CAD build for the part. Positions are in the model's coordinates, mm. Face numbers are marked on the shaded views. A direction names the side the tool comes from. Coordinates: 2 decimals unless noted, no trailing zeros. Order: outer loops, then holes, each group sorted by start corner. A loop starts at its lowest first (then second) coordinate and runs counter-clockwise, first axis right, second up.
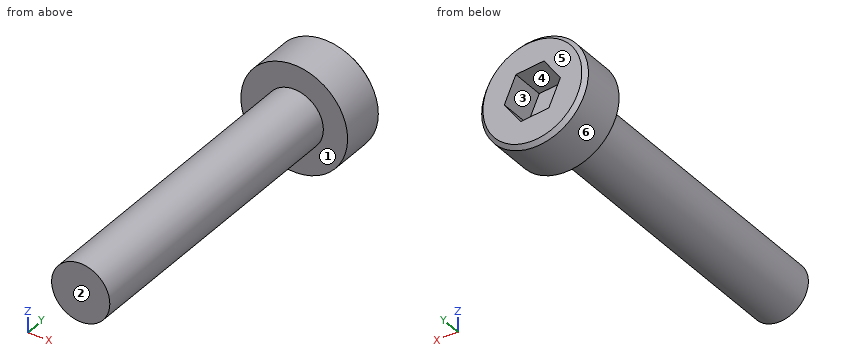
from build123d import *

# Parameters (mm, degrees)
F0_R     = 2.75
F1_DEPTH = 2.5
F3_DEPTH = 1.75
F4_SIZE  = 0.2
F5_R     = 1.5
F6_DEPTH = 16


with BuildPart() as f1:
    # F0 (on Front) → F1 (new body)
    with BuildSketch(Plane.XZ):
        Circle(F0_R)
    extrude(amount=F1_DEPTH)

    # F2 (on face) → F3 (cut)
    with BuildSketch(Plane(origin=(0, 0, 0), x_dir=(-1, 0, 0), z_dir=(0, 1, 0))):
        Polygon((1.446581, 0.145307), (0.597451, 1.325429), (-0.84913, 1.180122), (-1.446581, -0.145307), (-0.597451, -1.325429), (0.84913, -1.180122), align=None)
    extrude(amount=-F3_DEPTH, mode=Mode.SUBTRACT)

    # F4
    f4_edges = [f1.edges().sort_by_distance(p)[0] for p in [
        (-2.75, 0, 0),
    ]]
    chamfer(f4_edges, length=F4_SIZE)

    # F5 (on face) → F6 (join)
    with BuildSketch(Plane.XZ.offset(2.5)):
        Circle(F5_R)
    extrude(amount=F6_DEPTH)


solid = f1.part
1) Which spindle directions (+Z, -Z, +X, -X, +Y, -Y) get a long thin tool onto all of the face, cutting with end or side? Do the marked faces 1, 2 and 3. Say none if no direction does.
2) Slice it at C-C (y = -6.5). List the corners of the cut face in (x, z).
3) Slice it at A-A (y = -1.5). List the corners of the cut face in (x, z).
4) Two-plate mould, pull along X, no slides. Class the marked faces 4, 5 and 6: released by +X, released by -X, zero draft, split by the parting line, or undercut.
5) Slice it at B-B (x = 0). List the corners of the cut face in (y, z).
6) Drill centre lines: probe 1 along Y at (x, z) = (2, -1.5); probe 2 along X at (y, z) = (-14.25, -0.15); probe 3 along Z at (x, y) = (-1.1, -15.5). Where is each one in solid material? Low to high.
7) Pin check, flat tips, straight feed: P1, Ø0.8, axis at x = 0.5, z = -0.5, coming from the +Y side; P2, Ø2, axis at x = -2, y = -14, coming from the -Z side. Stop position of each tip, or through.
Worked out:
1. face 1: -Y
1. face 2: +Z, -Z, +X, -X, -Y
1. face 3: +Y
2. outline: circle Ø3 at (0, 0)
3. outline: circle Ø5.5 at (0, 0); hole (-1.45, 0.15) - (-0.85, -1.18) - (0.6, -1.33) - (1.45, -0.15) - (0.85, 1.18) - (-0.6, 1.33) - close
4. face 4: undercut
4. face 5: zero draft
4. face 6: split by the parting line
5. outline: (-18.5, -1.5) - (-2.5, -1.5) - (-2.5, -2.75) - (-0.2, -2.75) - (0, -2.55) - (0, -1.27) - (-1.75, -1.27) - (-1.75, 1.27) - (0, 1.27) - (0, 2.55) - (-0.2, 2.75) - (-2.5, 2.75) - (-2.5, 1.5) - (-18.5, 1.5) - close
6. probe 1: y = -2.5 to 0
6. probe 2: x = -1.49 to 1.49
6. probe 3: z = -1.02 to 1.02
7. P1: stops at y = -1.75
7. P2: stops at z = -1.12
